Autodesk Inventor part; units mm, degrees
ref_plane "YZ Plane" through (0, 0, 0) normal (1, 0, 0) x (0, 1, 0)
ref_plane "XZ Plane" through (0, 0, 0) normal (0, 1, 0) x (-1, 0, 0)
ref_plane "XY Plane" through (0, 0, 0) normal (0, 0, 1) x (1, 0, 0)
sketch "Sketch1" plane through (0, 0, 0) normal (0, 0, 1) x (1, 0, 0)
  circle A0 centre (0, 0) radius 94
  circle A1 centre (0, 0) radius 75
  line L0 (-13, 0) -> (-56, 22)
  line L1 (-130, 0) -> (137, 0) construction
  line L2 (0, 131.4545) -> (0, -117) construction
  line L3 (-13, 0) -> (-56, -22)
  line L4 (0, -131.4545) -> (0, 117) construction
  arc A2 (-56, 22) -> (-56, -22) centre (0, 0) ccw
  line L5 (13, 0) -> (56, 22)
  line L6 (13, 0) -> (56, -22)
  arc A3 (56, -22) -> (56, 22) centre (0, 0) ccw
  circle A4 centre (0, 0) radius 78.5
  dimension "d0" = 188
  dimension "d6" = 150
  dimension "d16" = 157
extrude "Extrusion1" add sketch "Sketch1" along normal blind 6.5 contours A0 | A4
extrude "Extrusion3" add sketch "Sketch1" along normal blind 8 contours A1
fillet "Fillet2" radius 2 1 edges at (-75, 0, 8)
chamfer "Chamfer1" distance 15 angle 15 1 edges at (-94, 0, 6.5) measured on face at (-71.1692, 50.8207, 6.5)
extrude "Extrusion4" add sketch "Sketch1" along normal blind 1 contours L3 A2 L0 | L5 A3 L6
fillet "Fillet3" radius 3 6 edges at (-60.1664, 0, 1) (-34.5, 11, 1) (-34.5, -11, 1) (34.5, 11, 1) (34.5, -11, 1) (60.1664, 0, 1)
extrude "Extrusion5" add sketch "Sketch1" against normal blind 15 contours A4
properties part number "hatch"
Part model, mm, in its own coordinate system. A direction names the side the tool comes from. Round coordinates to 2 decimals unless told otherwise and drop trailing zeros. Order: outer loops, then holes, each group sorted by start corner. A loop starts at its lowest first (then second) coordinate and runs counter-clockwise, first axis right, second up. Notation, with made-up numbers: (-18.75, 27) -> (-13.75, 27) arc R20 cw to (-13.75, 58) -> close; hole circle Ø4 at (46, 59). An arc over 180 degrees is marked (long way). Put each result on its own line as item: value.
Q1. Band-saw the part on A-A (x = 0). Give the cut face in (y, z).
From the geometry:
outline: (-94, 0) -> (-78.5, 0) -> (-78.5, -15) -> (-75, -15) -> (-75, 0) -> (75, 0) -> (75, -15) -> (78.5, -15) -> (78.5, 0) -> (94, 0) -> (94, 2.48) -> (79, 6.5) -> (75, 6.5) arc R2 ccw to (73.06, 8) -> (-73.06, 8) arc R2 ccw to (-75, 6.5) -> (-79, 6.5) -> (-94, 2.48) -> close
Q2. Wall check: line 1 (Y direction, x = 0, z = -6.5); line 2 (X direction, y = -68, z = -4.5); line 3 (Y direction, x = 5, z = -6.25). Give the ranges that are in metal, low to high. Write a range as [from, to].
From the geometry:
line 1: y = [-78.5, -75], [75, 78.5]
line 2: x = [-39.22, -31.64], [31.64, 39.22]
line 3: y = [-78.34, -74.83], [74.83, 78.34]
Q3. Pin check, flat tips, straight feed: pin 1 Ø4 at (x, y) = (48.5, -35) entering from -Z; pin 2 Ø1 at (y, z) = (61.5, -2.5) entering from +X; pin 3 Ø18 at (x, y) = (38.5, -6) entering from +Z; pin 4 Ø8 at (y, z) = (46.5, 4.5) entering from +X. Stop position of each tip, or through.
From the geometry:
pin 1: stops at z = 0
pin 2: stops at x = 49.41
pin 3: stops at z = 8
pin 4: stops at x = 83.56
Q4. Pull direction X, two halves, no side cores. Call faces 1 (the face through (-35.212, -10.351, 1.855)), 2 (the face through (-17.329, 78.037, 6.249)), 3 (the face through (70, -29, 6.5)): pulls with the +X half, pulls with the -X half, needs draft (parallel to the pull), parting line crosses it, or undercut.
From the geometry:
face 1: undercut
face 2: parting line crosses it
face 3: needs draft
Q5. Band-saw the part on B-B (z = -4.5). Give the cut face in (x, y), and give its area (3 significant figures).
From the geometry:
outline: circle Ø157 at (0, 0); hole circle Ø150 at (0, 0)
area: 1,690 mm2
Q6. Tool access for faces 4 (the face through (64, -40, -15)), 5 (the face through (-34.199, 10.846, 5.972)), 6 (the face through (-78.424, 3.451, -7.395)): list every direction of +Z, -Z, +X, -X, +Y, -Y with a clear straight run to the whole face (end or side of a thin tool).
From the geometry:
face 4: -Z, +X, -X, +Y, -Y
face 5: +Z
face 6: -Z
